Answer from the drawing. Dimensions are ordinates in mm from the lowest x, y and z of the part. Give positions to 0.01 mm unless a question says otherwise; leave off trailing zeros. Order: outer loops, then holes, each group sorted by start corner. A loop starts at its lowest first (then second) coordinate and runs counter-clockwise, first axis right, second up. Notation, with made-up numbers: (85.5, 62) - (134.5, 62) arc R20 ccw to (134.5, 94) - close; hole circle Ø7 at (25.5, -17.5). An arc over 180 degrees is marked (long way). Write each question's results on one line, items separated by ' | '.
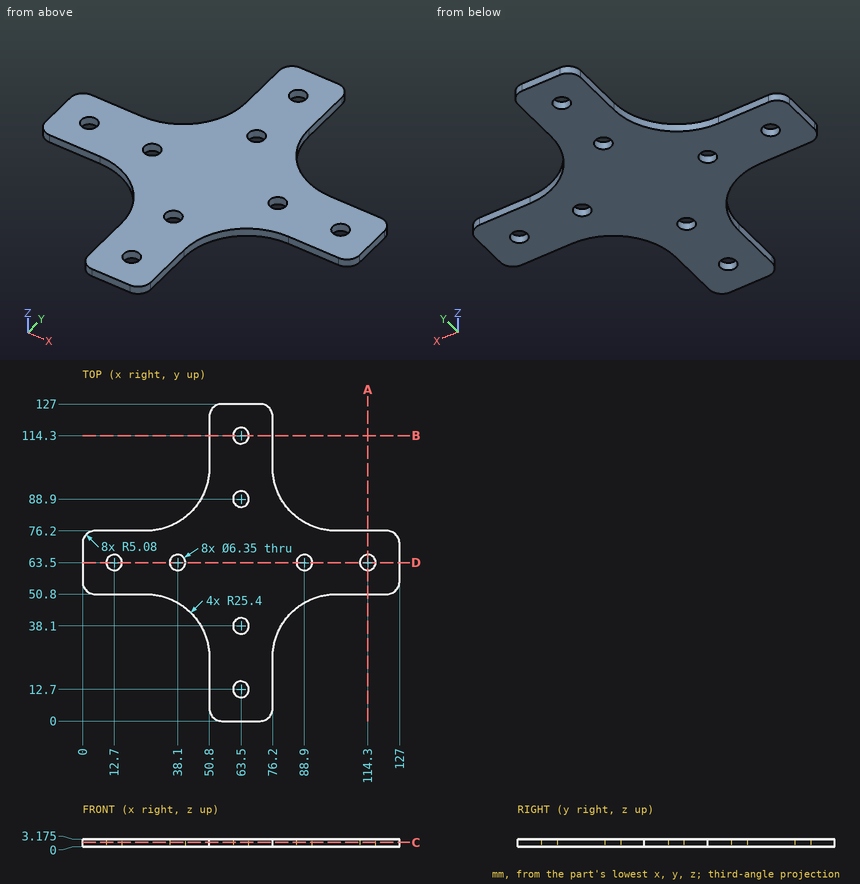
1. A cutting plane is placed at D-D, the plane y = 63.5. Write down the section's boundary in (x, z) (3 decimals), then the cut area to 3 significant figures.
Answer list:
outline: (0, 0) - (9.525, 0) - (9.525, 3.175) - (0, 3.175) - close; (15.875, 0) - (34.925, 0) - (34.925, 3.175) - (15.875, 3.175) - close; (41.275, 0) - (85.725, 0) - (85.725, 3.175) - (41.275, 3.175) - close; (92.075, 0) - (111.125, 0) - (111.125, 3.175) - (92.075, 3.175) - close; (117.475, 0) - (127, 0) - (127, 3.175) - (117.475, 3.175) - close | area: 323 mm^2
2. A cutting plane is placed at A-A, the plane x = 114.3. Write down the section's boundary in (y, z) (3 decimals).
Answer list:
outline: (50.8, 0) - (60.325, 0) - (60.325, 3.175) - (50.8, 3.175) - close; (66.675, 0) - (76.2, 0) - (76.2, 3.175) - (66.675, 3.175) - close
3. Straight lines are drawn through the part: line 1 (Y direction, x = 63.5, z = 1.4) (3 decimals); line 2 (X direction, y = 65.5, z = 0.4); line 3 (Y direction, x = 114.3, z = 1.3) (3 decimals). For each, find the intervals that lie inside material, in ascending order. Write a range as [from, to].
Answer list:
line 1: [0, 9.525], [15.875, 34.925], [41.275, 85.725], [92.075, 111.125], [117.475, 127] | line 2: [0, 10.23], [15.17, 35.63], [40.57, 86.43], [91.37, 111.83], [116.77, 127] | line 3: [50.8, 60.325], [66.675, 76.2]
4. A cutting plane is placed at C-C, the plane z = 1.85. State how many separate pieces and enclosed holes the cut face has, then the cut area to 3 significant figures.
Answer list:
separate pieces: 1 | enclosed holes: 8 | area: 6,060 mm^2
5. Given P1, Ø1, axis at y = 16.5, z = 1.5, coming from the +X side; P2, Ø1.6, axis at x = 110.5, z = 1.5, coming from the +Y side; P3, Ø1.5, axis at y = 102, z = 1.5, coming from the -X side; P4, Ø8.5, axis at x = 88.9, y = 63.5, coming from the +Z side (3 decimals), each flat-ended and moving along its own axis, determine where each tip first touches the part or whether it passes through.
Answer list:
P1: x = 76.2 | P2: y = 76.2 | P3: x = 50.8 | P4: z = 3.175
